```python
from build123d import *


with BuildPart() as f1:
    # F0 (on Front) → F1 (revolve)
    with BuildSketch(Plane.XZ):
        with BuildLine():
            Line((0, 30), (0, 84))
            Line((0, 84), (-24, 84))
            Line((-24, 84), (-24, 67.5))
            Line((-24, 67.5), (-14, 67.5))
            ThreePointArc((-14, 67.5), (-12.585786, 66.914214), (-12, 65.5))
            Line((-12, 65.5), (-12, 46))
            ThreePointArc((-12, 46), (-12.585786, 44.585786), (-14, 44))
            Line((-14, 44), (-24, 44))
            Line((-24, 44), (-24, 34))
            Line((-24, 34), (-20.694984, 34))
            Line((-20.694984, 34), (-20.694984, 35.5))
            Line((-20.694984, 35.5), (-17.731871, 35.5))
            Line((-17.731871, 35.5), (-17.731871, 34))
            Line((-17.731871, 34), (-3, 34))
            Line((-3, 34), (-3, 30))
            Line((-3, 30), (0, 30))
        make_face()
        with BuildLine():
            Line((24, 84), (0, 84))
            Line((0, 84), (0, 30))
            Line((0, 30), (3, 30))
            Line((3, 30), (3, 34))
            Line((3, 34), (17.731871, 34))
            Line((17.731871, 34), (17.731871, 35.5))
            Line((17.731871, 35.5), (20.694984, 35.5))
            Line((20.694984, 35.5), (20.694984, 34))
            Line((20.694984, 34), (24, 34))
            Line((24, 34), (24, 44))
            Line((24, 44), (14, 44))
            ThreePointArc((14, 44), (12.585786, 44.585786), (12, 46))
            Line((12, 46), (12, 65.5))
            ThreePointArc((12, 65.5), (12.585786, 66.914214), (14, 67.5))
            Line((14, 67.5), (24, 67.5))
            Line((24, 67.5), (24, 84))
        make_face()
    revolve(axis=Axis((-12, 0, 0), (-1, 0, 0)))


solid = f1.part
```
Input: part model. Units: mm. Frame: model coordinates. A direction names the side the tool comes from. Give positions to 0.01 mm unless a question says otherwise; leave off trailing zeros. Write each loop counter-clockwise with the first axis right and the second up, starting at its lowest first coordinate (ties: lowest second). Pieces come first, ordered by that corner, then holes. Notation, with made-up numbers: (-31.5, 65) - (20.5, 65) arc R12 ccw to (20.5, 83) - close; hole circle Ø7 at (76, -30). An arc over 180 degrees is marked (long way). Write item = value, one per line. Start each with the question number.
1. Mould query, pull axis Y, two halves, no side actions, for faces 6 (the flat face through (-12, -14, -45)), 7 (the flat face through (24, -26, -23)), 8 (the flat face through (12, -14, 45)), 9 (the cylindrical face through (-0.34, 25.23, 80.12)). Classes: released by +Y, released by -Y, zero draft, split by the parting line, or undercut.
2. First-contact query: pin 1 Ø10 at (x, z) = (-8.5, -54.5) entering from -Y; pin 2 Ø8 at (x, z) = (-5, -65.5) entering from -Y; pin 3 Ø8 at (x, z) = (1.5, -17) entering from -Y. Flat tips, straight axial feed; report the tip coordinate or a pass-through.
3. Access query for faces 1 (the flat face through (24, 69, 0)), 2 (the cylindrical face through (19.234, -34.656, -7.696)), 3 (the cylindrical face through (0.04, 1.32, -29.97)), 4 (the cylindrical face through (22.37, 28.67, 18.28)), 5 (the cylindrical face through (-22.32, 28.67, 18.28)). Directions: +Z, -Z, +X, -X, +Y, -Y. A direction counts if a zero-diameter tool reaches every point of the face in a straight line with its end or side. Return the directions, or none.
4. Ray query, L1, parallel to X at y = -2.5, z = -34; L2, parallel to Y at x = -18, z = 0; L3, parallel to Y at x = -1.15, z = 0. Return the intervals inside material, ascending.
5. Section query A-A, the plane x = 1. Output: boundary loops of the cut face in (y, z).
Check sheet entries:
q1.face_6 = undercut
q1.face_7 = zero draft
q1.face_8 = undercut
q1.face_9 = split by the parting line
q2.pin_1 = -67.87
q2.pin_2 = -57.22
q2.pin_3 = -82.99
q3.face_1 = +Z, -Z, +X, +Y, -Y
q3.face_2 = none
q3.face_3 = +X, -X
q3.face_4 = +X
q3.face_5 = -X
q4.L1 = -24 to -20.69, -17.73 to 17.73, 20.69 to 24
q4.L2 = -84 to -67.5, -44 to -35.5, 35.5 to 44, 67.5 to 84
q4.L3 = -84 to -30, 30 to 84
q5.outline = circle Ø168 at (0, 0); hole circle Ø60 at (0, 0)
